from build123d import *

# Parameters (mm, degrees)
SKETCH_1_R               = 78
EXTRUDE_1_DEPTH          = 8
SKETCH_2_R               = 50.8
EXTRUDE_2_DEPTH          = 252
SKETCH_3_R               = 50
EXTRUDE_3_DEPTH          = 282
CUT_EXTRUDE_1_DEPTH      = 303.806869143
CUT_EXTRUDE_1_DEPTH_BACK = 303.806869143
SKETCH_4_R               = 41.8
SKETCH_6_R               = 45
CUT_EXTRUDE_3_DEPTH      = 10
CUT_EXTRUDE_START        = -10
SKETCH_7_R               = 45
CUT_EXTRUDE_4_DEPTH      = 10
CUT_EXTRUDE_5_DEPTH      = 303.806869143
CUT_EXTRUDE_5_DEPTH_BACK = 303.806869143
SKETCH_8_R               = 4.5
CHAMFER_1_SIZE           = 0.5
CHAMFER_2_SIZE           = 0.5


with BuildPart() as part:
    # ｽｹｯﾁ1 → ﾎﾞｽ - 押し出し1 (new body)
    with BuildSketch(Plane(origin=(0, 0, 0), x_dir=(0, 0, -1), z_dir=(1, 0, 0))):
        Circle(SKETCH_1_R)
    extrude(amount=EXTRUDE_1_DEPTH)

    # ｽｹｯﾁ2 → ﾎﾞｽ - 押し出し2 (add)
    with BuildSketch(Plane(origin=(0, 0, 0), x_dir=(0, 0, -1), z_dir=(1, 0, 0))):
        Circle(SKETCH_2_R)
    extrude(amount=EXTRUDE_2_DEPTH)

    # ｽｹｯﾁ3 → ﾎﾞｽ - 押し出し3 (add)
    with BuildSketch(Plane(origin=(0, 0, 0), x_dir=(0, 0, -1), z_dir=(1, 0, 0))):
        Circle(SKETCH_3_R)
    extrude(amount=EXTRUDE_3_DEPTH)

    # ｽｹｯﾁ4 → ｶｯﾄ - 押し出し1 (cut, two sides: drawn at the far end of the back side and taken through both)
    with BuildSketch(Plane(origin=(0, 0, 0), x_dir=(0, 0, -1), z_dir=(1, 0, 0)).offset(-CUT_EXTRUDE_1_DEPTH_BACK)):
        Circle(SKETCH_4_R)
    extrude(amount=CUT_EXTRUDE_1_DEPTH + CUT_EXTRUDE_1_DEPTH_BACK, mode=Mode.SUBTRACT)

    # ｽｹｯﾁ6 → ｶｯﾄ - 押し出し3 (cut)
    with BuildSketch(Plane(origin=(0, 0, 0), x_dir=(0, 0, -1), z_dir=(1, 0, 0))):
        Circle(SKETCH_6_R)
    extrude(amount=CUT_EXTRUDE_3_DEPTH, mode=Mode.SUBTRACT)

    # ｽｹｯﾁ7 → ｶｯﾄ - 押し出し4 (cut)
    with BuildSketch(Plane(origin=(282, 0, 0), x_dir=(0, 0, -1), z_dir=(1, 0, 0)).offset(CUT_EXTRUDE_START)):
        Circle(SKETCH_7_R)
    extrude(amount=CUT_EXTRUDE_4_DEPTH, mode=Mode.SUBTRACT)

    # ｽｹｯﾁ8 → ｶｯﾄ - 押し出し5 (cut, two sides: drawn at the far end of the back side and taken through both)
    with BuildSketch(Plane(origin=(0, 0, 0), x_dir=(0, 0, -1), z_dir=(1, 0, 0)).offset(-CUT_EXTRUDE_5_DEPTH_BACK)):
        with Locations((-68.5, 0)):
            Circle(SKETCH_8_R)
        with Locations((34.25, 59.322740159)):
            Circle(SKETCH_8_R)
        with Locations((34.25, -59.322740159)):
            Circle(SKETCH_8_R)
    extrude(amount=CUT_EXTRUDE_5_DEPTH + CUT_EXTRUDE_5_DEPTH_BACK, mode=Mode.SUBTRACT)

    # 面取り1
    chamfer_1_edges = [part.edges().sort_by_distance(p)[0] for p in [
        (0, 0, 45),
    ]]
    chamfer(chamfer_1_edges, length=CHAMFER_1_SIZE)

    # 面取り2
    chamfer_2_edges = [part.edges().sort_by_distance(p)[0] for p in [
        (282, 0, 45),
    ]]
    chamfer(chamfer_2_edges, length=CHAMFER_2_SIZE)


solid = part.part
The listing builds one solid part. Answer for the finished solid, in the listing's coordinates (mm). A direction names the side the tool comes from. Round coordinates to 2 decimals unless told otherwise and drop trailing zeros. Write each loop counter-clockwise with the first axis right and the second up, starting at its lowest first coordinate (ties: lowest second). Pieces come first, ordered by that corner, then holes. Notation, with made-up numbers: (88.5, 65) - (147.5, 65) arc R25 cw to (147.5, 77) - close; hole circle Ø8 at (-12.5, 3). An arc over 180 degrees is marked (long way). Use a Markdown table: item, result. Add a question column.
1. Consider line 1 (Y direction, x = 279, z = 0); line 2 (Y direction, x = 3.25, z = -34.25); line 3 (Y direction, x = 4, z = 0). Determine where each line is inside the solid, lowest interval first.
2. The part is cut by section A-A (y = 0). Give the number of separate pieces and of enclosed holes in the cut face, and give its area (3 significant figures).
3. Flat-ended cylindrical pins translate along their axes: P1, Ø4, axis at x = 111.5, y = 46.5, coming from the -Z side; P2, Ø1, axis at x = 220.5, z = 27.5, coming from the +Y side; P3, Ø5, axis at x = 42.5, y = -45.5, coming from the +Z side. Find the tip coordinate at first contact, or state that the pin passes through.
4. For a pull along Y with two mould halves and no side action, classify faces 1 (the face through (128.292, -49.592, 11.012)), 2 (the face through (10, -40, -13)), 3 (the face through (0, -34, -34)) as +Y half, -Y half, draft (parallel to the pull), parting line (faces both ways), or undercut.
5. The part is cut by section C-C (x = 255). Write down the section's boundary in (y, z), and give its area (3 significant figures).
6. The part is cut by section D-D (z = 68.5). Write down the section's boundary in (x, y), and give its area (3 significant figures).
7. The part is cut by section B-B (z = 0). Write down the section's boundary in (x, y), and give its area (3 significant figures).
8. A tool of negligible diameter and unlimited length cuts with its end or side. For faces 4 (the face through (282, -41, -22)), 5 (the face through (5.184, -39.923, -20.765)), 6 (the face through (266.79, 15.02, -47.69)), from which of +Z, -Z, +X, -X, +Y, -Y can it reach the whole face along a straight path? Write none if from no direction.
Reported:
| question | item | result |
|---|---|---|
| 1 | line 1 | -50 to -45, 45 to 50 |
| 1 | line 2 | -70.08 to -63.82, -54.82 to -29.19, 29.19 to 54.82, 63.82 to 70.08 |
| 1 | line 3 | -78 to -45, 45 to 78 |
| 2 | separate pieces | 3 |
| 2 | enclosed holes | 0 |
| 2 | area | 5,260 mm^2 |
| 3 | P1 | z = -24.5 |
| 3 | P2 | y = 43.03 |
| 3 | P3 | z = 27.05 |
| 4 | face 1 | parting line |
| 4 | face 2 | undercut |
| 4 | face 3 | draft |
| 5 | outline | circle Ø100 at (0, 0); hole circle Ø83.6 at (0, 0) |
| 5 | area | 2,360 mm^2 |
| 6 | outline | (0, -37.31) - (8, -37.31) - (8, -4.5) - (0, -4.5) - close; (0, 4.5) - (8, 4.5) - (8, 37.31) - (0, 37.31) - close |
| 6 | area | 525 mm^2 |
| 7 | outline | (0, -78) - (8, -78) - (8, -50.8) - (252, -50.8) - (252, -50) - (282, -50) - (282, -45.5) - (281.5, -45) - (272, -45) - (272, -41.8) - (10, -41.8) - (10, -45) - (0.5, -45) - (0, -45.5) - close; (0, 45.5) - (0.5, 45) - (10, 45) - (10, 41.8) - (272, 41.8) - (272, 45) - (281.5, 45) - (282, 45.5) - (282, 50) - (252, 50) - (252, 50.8) - (8, 50.8) - (8, 78) - (0, 78) - close |
| 7 | area | 5,330 mm^2 |
| 8 | face 4 | +Z, -Z, +X, +Y, -Y |
| 8 | face 5 | -X |
| 8 | face 6 | +X |
